Source: CAD feature listing. Evaluate the final solid. Frame: model axes, mm. A direction names the side the tool comes from. Round coordinates to 2 decimals unless told otherwise and drop trailing zeros. Order: outer loops, then holes, each group sorted by start corner. A loop starts at its lowest first (then second) coordinate and runs counter-clockwise, first axis right, second up. Notation, with made-up numbers: (17.25, 20.25) -> (51.25, 20.25) arc R32 ccw to (51.25, 46.25) -> close; hole circle Ø10 at (8, 25.25). An arc over 180 degrees is marked (long way). One line per item, written item: value. Start each with the question number.
1) Section C-C (x = -54). Return the cut outline in (y, z).
2) Ray query, L1, parallel to Z at x = 29, y = 4.7; L2, parallel to X at y = 1.5, z = -40; L3, parallel to Z at x = -46.5, y = 2.6. Return the intervals inside material, ascending.
3) Pin query (flat end, axial travel): P1, Ø7, axis at x = 40, z = -40, coming from the -Y side; P2, Ø1.5, axis at x = -0.5, y = 0.5, coming from the -Z side. Return the tip coordinate at first contact, or that it passes through.
4) Reachability of faces 1 (the face through (-60, 2, 54)), 2 (the face through (-6, 2, -12)), 3 (the face through (53, 2, -60)) from +Z, -Z, +X, -X, +Y, -Y: full face, straight path, thin tool, end or side. Return the list, or none.
5) Section A-A (x = 50). Return the cut outline in (y, z), and give its area (3 significant figures).
6) Mould query, pull axis Z, two halves, no side actions, for faces 4 (the face through (0, 2, -60)), 5 (the face through (60, 2, -1)), 6 (the face through (-38.19, 2.46, 41.16)), 7 (the face through (-75, 2, 30)). Classes: pulls with the +Z half, pulls with the -Z half, needs draft (parallel to the pull), parting line crosses it, or undercut.
7) Section B-B (z = 40). Return the cut outline in (x, y), and give its area (3 significant figures).
8) Section D-D (y = 2.65). State how many separate pieces and enclosed holes the cut face has, and give its area (3 significant figures).
```python
from build123d import *

# Parameters (mm, degrees)
SKETCH1_R           = 2.15
SKETCH1_W           = 12
SKETCH1_H           = 5
BOSS_EXTRUDE1_DEPTH = 5
FILLET1_R           = 2
FILLET2_R           = 1


with BuildPart() as part:
    # Sketch1 → Boss-Extrude1 (new body)
    with BuildSketch(Plane(origin=(0, 0, 0), x_dir=(1, 0, 0), z_dir=(0, 1, 0))):
        with BuildLine():
            Line((60, -60), (-60, -60))
            Line((-60, -60), (-60, -45))
            ThreePointArc((-60, -45), (-75, -30), (-60, -15))
            Line((-60, -15), (-60, 15))
            ThreePointArc((-60, 15), (-45, 30), (-60, 45))
            Line((-60, 45), (-60, 60))
            Line((-60, 60), (-45, 60))
            ThreePointArc((-45, 60), (-30, 75), (-15, 60))
            Line((-15, 60), (15, 60))
            ThreePointArc((15, 60), (30, 45), (45, 60))
            Line((45, 60), (60, 60))
            Line((60, 60), (60, -60))
        make_face()
        with Locations(Location((-40, 40, 0), (0, 0, 270))):
            Circle(SKETCH1_R, mode=Mode.SUBTRACT)
        with Locations(Location((40, 40, 0), (0, 0, 270))):
            Circle(SKETCH1_R, mode=Mode.SUBTRACT)
        with Locations(Location((40, -40, 0), (0, 0, 270))):
            Circle(SKETCH1_R, mode=Mode.SUBTRACT)
        with Locations(Location((-40, -40, 0), (0, 0, 270))):
            Circle(SKETCH1_R, mode=Mode.SUBTRACT)
        with Locations(Location((30, 12, 0), (0, 0, 270))):
            Circle(SKETCH1_R, mode=Mode.SUBTRACT)
        with Locations(Location((50, 12, 0), (0, 0, 270))):
            Circle(SKETCH1_R, mode=Mode.SUBTRACT)
        with Locations(Location((30, -12, 0), (0, 0, 270))):
            Circle(SKETCH1_R, mode=Mode.SUBTRACT)
        with Locations(Location((50, -12, 0), (0, 0, 270))):
            Circle(SKETCH1_R, mode=Mode.SUBTRACT)
        with Locations(Location((0, 40, 0), (0, 0, 270))):
            Circle(SKETCH1_R, mode=Mode.SUBTRACT)
        with Locations(Location((0, -40, 0), (0, 0, 270))):
            Circle(SKETCH1_R, mode=Mode.SUBTRACT)
        with Locations((0, 12)):
            Rectangle(SKETCH1_W, SKETCH1_H, mode=Mode.SUBTRACT)
    extrude(amount=BOSS_EXTRUDE1_DEPTH)

    # Fillet1
    fillet1_edges = [part.edges().sort_by_distance(p)[0] for p in [
        (-45, 2.5, -60),
        (-15, 2.5, -60),
        (15, 2.5, -60),
        (45, 2.5, -60),
        (-60, 2.5, 45),
        (-60, 2.5, 15),
        (-60, 2.5, -15),
        (-60, 2.5, -45),
    ]]
    fillet(fillet1_edges, radius=FILLET1_R)

    # Fillet2
    fillet2_edges = [part.edges().sort_by_distance(p)[0] for p in [
        (-6, 2.5, -14.5),
        (-6, 2.5, -9.5),
        (6, 2.5, -9.5),
        (6, 2.5, -14.5),
    ]]
    fillet(fillet2_edges, radius=FILLET2_R)


solid = part.part
```
Findings:
1. outline: (0, -60) -> (5, -60) -> (5, -43.75) -> (0, -43.75) -> close; (0, -16.25) -> (5, -16.25) -> (5, 60) -> (0, 60) -> close
2. L1: -45.03 to -13.9, -10.1 to 10.1, 13.9 to 60
2. L2: -48.82 to -42.15, -37.85 to -2.15, 2.15 to 37.85, 42.15 to 60
2. L3: -60.04 to -36.54, -23.46 to 60
3. P1: y = 0
3. P2: z = -60
4. face 1: +Z, -X, +Y, -Y
4. face 2: +Y, -Y
4. face 3: -Z, +X, +Y, -Y
5. outline: (0, -60) -> (5, -60) -> (5, -14.15) -> (0, -14.15) -> close; (0, -9.85) -> (5, -9.85) -> (5, 9.85) -> (0, 9.85) -> close; (0, 14.15) -> (5, 14.15) -> (5, 60) -> (0, 60) -> close
5. area: 557 mm2
6. face 4: pulls with the -Z half
6. face 5: needs draft
6. face 6: undercut
6. face 7: parting line crosses it
7. outline: (-71.18, 0) -> (-42.15, 0) -> (-42.15, 5) -> (-71.18, 5) -> close; (-37.85, 0) -> (-2.15, 0) -> (-2.15, 5) -> (-37.85, 5) -> close; (2.15, 0) -> (37.85, 0) -> (37.85, 5) -> (2.15, 5) -> close; (42.15, 0) -> (60, 0) -> (60, 5) -> (42.15, 5) -> close
7. area: 591 mm2
8. separate pieces: 1
8. enclosed holes: 11
8. area: 14,200 mm2
